The listing builds one solid part. Answer for the finished solid, in the listing's coordinates (mm). Face numbers are marked on the shaded views. Give positions to 0.01 mm unless a question says otherwise; leave off trailing zeros. Order: outer loops, then holes, each group sorted by start corner. A loop starts at its lowest first (then second) coordinate and runs counter-clockwise, first axis right, second up.
```python
from build123d import *

# Parameters (mm, degrees)
BOSS_EXTRU_1_DEPTH      = 3.5
ESQUISSE2_W             = 4
ESQUISSE2_H             = 4
ENL_V_MAT_EXTRU_1_DEPTH = 2.9
CONG_1_R                = 2


with BuildPart() as part:
    # Esquisse1 → Boss.-Extru.1 (new body)
    with BuildSketch(Plane.XY):
        Polygon((-12.45, 0), (12.45, 0), (0, 21.564032554), align=None)
    extrude(amount=BOSS_EXTRU_1_DEPTH)

    # Esquisse2 → Enlèv. mat.-Extru.1 (cut)
    with BuildSketch(Plane(origin=(0, 0, 0), x_dir=(-1, 0, 0), z_dir=(0, 0, -1))):
        with Locations((0, 5.874833395)):
            Rectangle(ESQUISSE2_W, ESQUISSE2_H)
    extrude(amount=-ENL_V_MAT_EXTRU_1_DEPTH, mode=Mode.SUBTRACT)

    # Congé1
    cong_1_edges = [part.edges().sort_by_distance(p)[0] for p in [
        (0, 21.564032554, 1.75),
        (12.45, 0, 1.75),
        (-12.45, 0, 1.75),
    ]]
    fillet(cong_1_edges, radius=CONG_1_R)


solid = part.part
```
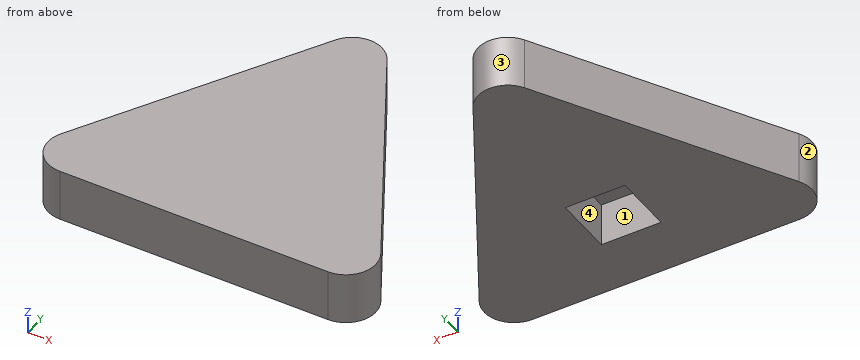
1) Find section C-C (y = 6.25). Write down the section's boundary in (x, z).
Geometry says:
outline: (-8.84, 0) - (-2, 0) - (-2, 2.9) - (2, 2.9) - (2, 0) - (8.84, 0) - (8.84, 3.5) - (-8.84, 3.5) - close
2) Find section D-D (x = -8.25). Write down the section's boundary in (y, z), then the cut area to 3 significant figures.
Geometry says:
outline: (0, 0) - (7.27, 0) - (7.27, 3.5) - (0, 3.5) - close
area: 25.5 mm2
3) For a pull along Y with two mould halves and no side action, classify the marked faces 1, 2, 3 and 4 as +Y half, -Y half, draft (parallel to the pull), parting line (faces both ways), or undercut.
Geometry says:
face 1: undercut
face 2: parting line
face 3: +Y half
face 4: undercut
4) Find section A-A (z = 2.4). Write down the section's boundary in (x, y).
Geometry says:
outline: (-10.72, 3) arc R2 ccw to (-8.99, 0) - (8.99, 0) arc R2 ccw to (10.72, 3) - (1.73, 18.56) arc R2 ccw to (-1.73, 18.56) - close; hole (-2, 3.87) - (2, 3.87) - (2, 7.87) - (-2, 7.87) - close
5) Straight lines are drawn through the part: probe 1 along Y at (x, z) = (0.5, 2.6); probe 2 along Y at (x, z) = (-1, 1.35); probe 3 along X at (y, z) = (12.75, 1.55). For each, find the intervals that lie inside material, in ascending order.
Geometry says:
probe 1: y = 0 to 3.87, 7.87 to 19.5
probe 2: y = 0 to 3.87, 7.87 to 19.3
probe 3: x = -5.09 to 5.09
6) Find section B-B (x = 0). Write down the section's boundary in (y, z).
Geometry says:
outline: (0, 0) - (3.87, 0) - (3.87, 2.9) - (7.87, 2.9) - (7.87, 0) - (19.56, 0) - (19.56, 3.5) - (0, 3.5) - close
7) Given P1, Ø1, axis at x = -4.5, z = 2.5, coming from the +Y side; P2, Ø1.4, axis at x = 1, z = 1, coming from the +Y side; P3, Ø1, axis at x = 5.5, z = 1.5, coming from the +Y side, each flat-ended and moving along its own axis, determine where each tip first touches the part or whether it passes through.
Geometry says:
P1: stops at y = 14.64
P2: stops at y = 19.54
P3: stops at y = 12.9
